Here's how the part is built. I have some questions about the finished solid (model axes, mm). A direction names the side the tool comes from. Coordinates: 2 decimals unless noted, no trailing zeros. Write each loop counter-clockwise with the first axis right and the second up, starting at its lowest first coordinate (ties: lowest second). Pieces come first, ordered by that corner, then holes.
(1) Please list where these lines run through material, in increasing order: probe 1 along Y at (x, z) = (-6.5, -21.5); probe 2 along Y at (x, z) = (17, -14.5); probe 3 along Z at (x, y) = (-0.5, -26).
(2) Imagine slicing it at A-A, the plane z = 0. List the corners of the cut face in (x, y) for me.
(3) Imagine slicing it at D-D, the plane x = -21. State how many separate pieces and enclosed holes the cut face has, plus the area to 3 significant figures.
(4) Which directions (+Z, -Z, +X, -X, +Y, -Y) give clear straight access to the entire face, cutting with the end or side of a thin tool? Please do faces 1 (the cylindrical face through (-23.846, -32.535, -7.509)), 2 (the conical face through (3.387, -20.626, 15.254)).
(5) For pin 1 Ø10 at (x, y) = (-8, -20) entering from -Z; pin 2 Ø1.5 at (y, z) = (-9.5, -6.5) entering from +X; pin 3 Ø1 at (x, y) = (-15, 23) entering from -Z, each with a flat end and sliding along its axis, tell me the tip position at first contact or that it passes through.
(6) Thinking about a two-plate mould opening in Y: for faces 3 (the flat face through (0, 35, 0)), 4 (the cylindrical face through (-23.846, 32.535, -7.509)), 5 (the flat face through (0, -35, 0)), 6 (the conical face through (3.387, 20.626, 15.254)), which applies, released by +Y, released by -Y, zero draft, split by the parting line, or undercut?
(7) Imagine slicing it at C-C, the plane y = 21. List the corners of the cut face in (x, z) for me, plus the area to 3 significant figures.
(8) Imagine slicing it at B-B, the plane x = 0. List the corners of the cut face in (y, z) for me.
```python
from build123d import *


with BuildPart() as part:
    # 草图1 → 旋转2 (revolve)
    with BuildSketch(Plane.XY):
        with BuildLine():
            Line((0, 20), (0, -20))
            Line((0, -20), (15, -20))
            ThreePointArc((15, -20), (25, 0), (15, 20))
            Line((15, 20), (0, 20))
        make_face()
    revolve(axis=Axis((0, 20, 0), (0, -1, 0)))

    # 草图2 → 旋转3 (revolve)
    with BuildSketch(Plane.XY, mode=Mode.PRIVATE) as revolve_3_sk:
        Polygon((0, 20), (15, 20), (25, 30), (25, 35), (0, 35), align=None)
    revolve_3 = revolve(revolve_3_sk.sketch.rotate(Axis((0, 35, 0), (0, -1, 0)), 180), axis=Axis((0, 35, 0), (0, -1, 0)))

    # 镜向1: 旋转3 across plane
    add(revolve_3.mirror(Plane.ZX))


solid = part.part
```
Recorded:
1. probe 1: y = -35 to -27.46, -10.98 to 10.98, 27.46 to 35
1. probe 2: y = -35 to -27.34, -11.21 to 11.21, 27.34 to 35
1. probe 3: z = -20.99 to 20.99
2. outline: (-25, -35) - (25, -35) - (25, -30) - (15, -20) arc R25 ccw to (15, 20) - (25, 30) - (25, 35) - (-25, 35) - (-25, 30) - (-15, 20) arc R25 ccw to (-15, -20) - (-25, -30) - close
3. separate pieces: 3
3. enclosed holes: 0
3. area: 991 mm2
4. face 1: +Y, -Y
4. face 2: none
5. pin 1: stops at z = -18.75
5. pin 2: stops at x = 22.57
5. pin 3: stops at z = -11.07
6. face 3: released by +Y
6. face 4: zero draft
6. face 5: released by -Y
6. face 6: undercut
7. outline: circle Ø32 at (0, 0)
7. area: 804 mm2
8. outline: (-35, -25) - (-30, -25) - (-20, -15) arc R25 ccw to (20, -15) - (30, -25) - (35, -25) - (35, 25) - (30, 25) - (20, 15) arc R25 ccw to (-20, 15) - (-30, 25) - (-35, 25) - close
